Check sheet for the drawn part. Datum: minimum x, y, z corner. Units: mm. Give positions to 0.01 mm unless a question says otherwise; leave off trailing zeros. Order: outer loops, then holes, each group sorted by start corner. A loop starts at its lowest first (then second) coordinate and runs counter-clockwise, first axis right, second up. Notation, with made-up numbers: M 89.25,37 L 98.25,37 A16 ccw 98.25,44 Z; hole C 70.5,-5 d5. An arc over 180 degrees is marked long. One line per question, with ' | ' between items. Start each with the question number.
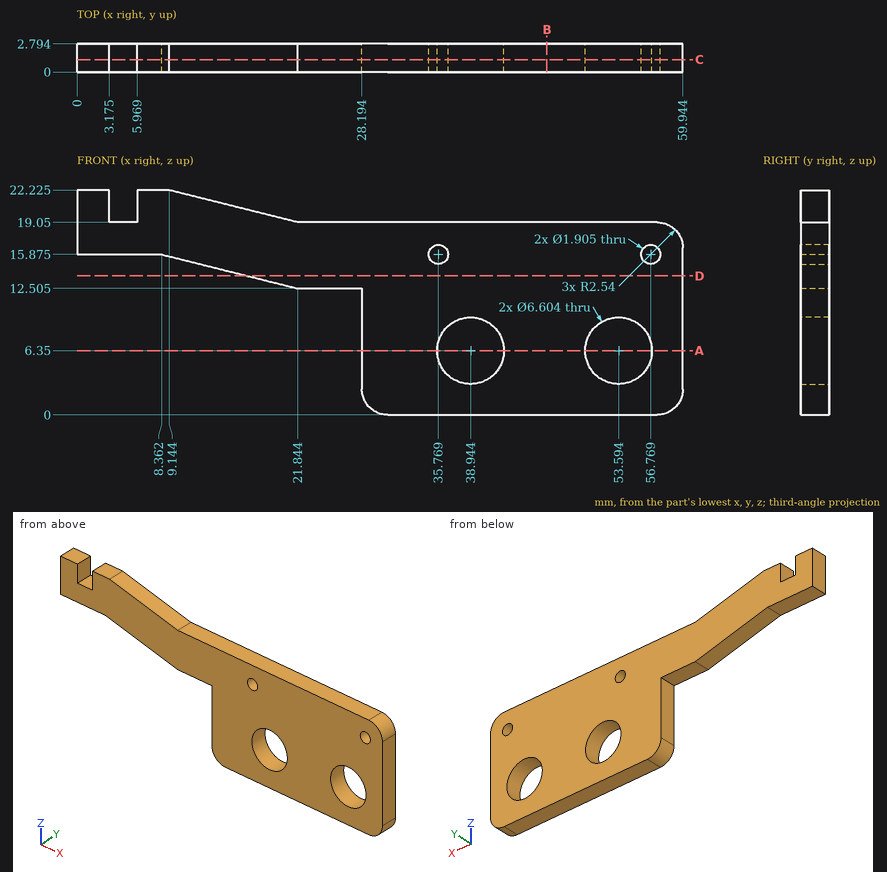
Item 1: Section check B-B, the plane x = 46.5. Record the cut outline in (y, z).
Item 2: Section check D-D, the plane z = 13.75. Record the cut outline in (x, y), then the cut area to 3 significant figures.
Item 3: Section check C-C, the plane y = 1.25. State how many separate pieces and enclosed holes the cut face has.
Item 4: Go/stop test with flat-tipped pins: P1, Ø0.8, axis at x = 45.5, y = 2, coming from the +Z side; P2, Ø1, axis at x = 15, y = 2, coming from the -Z side; P3, Ø4, axis at x = 53.594, z = 6.35, coming from the +Y side; P4, Ø1.4, axis at x = 6, y = 2, coming from the -Z side (3 decimals). Record where each tip stops, or that it passes through.
Item 5: Scan lines: probe 1 along X at (y, z) = (2.65, 16) (1 decimal); probe 2 along X at (y, z) = (1.8, 6.35); probe 3 along Z at (x, y) = (39, 1.85). Record each from-to range of solid material in increasing order. Write a range as [from, to].
Item 6: Section check A-A, the plane z = 6.35. Record the cut outline in (x, y).
Reported:
1) outline: M 0,0 L 2.79,0 L 2.79,19.05 L 0,19.05 Z
2) outline: M 16.86,0 L 59.94,0 L 59.94,2.79 L 16.86,2.79 Z | area: 120 mm^2
3) separate pieces: 1 | enclosed holes: 4
4) P1: stops at z = 19.05 | P2: stops at z = 14.09 | P3: passes through | P4: stops at z = 15.875
5) probe 1: x = [0, 34.8], [36.7, 55.8], [57.7, 59.9] | probe 2: x = [28.19, 35.64], [42.25, 50.29], [56.9, 59.94] | probe 3: z = [0, 3.05], [9.65, 19.05]
6) outline: M 28.19,0 L 35.64,0 L 35.64,2.79 L 28.19,2.79 Z; M 42.25,0 L 50.29,0 L 50.29,2.79 L 42.25,2.79 Z; M 56.9,0 L 59.94,0 L 59.94,2.79 L 56.9,2.79 Z
